Geometry: final body of the model. Coordinates: model frame, mm. Face numbers are marked on the shaded views. A direction names the side the tool comes from. Round coordinates to 2 decimals unless told otherwise and drop trailing zeros. Loops run counter-clockwise (first coordinate to the right, second up) from the corner with the lowest first, then second, coordinate; pieces in that order, holes last. Notation, with made-up numbers: (9, 36.25) - (35, 36.25) arc R31 cw to (35, 70.25) - close; hole circle Ø7 at (41.5, 45). An arc over 180 degrees is marked (long way). Answer as a JSON object with one key per item and string values. Group by question number.
Item 1: Section B-B (y = 15). Return the cut outline in (x, z), plus the area to 3 significant figures.
Item 2: Line query: line 1 (Y direction, x = -51.5, z = -28); line 2 (Z direction, x = -10, y = 16.5); line 3 (Z direction, x = -20, y = 8.5). Output: solid intervals per line, ascending.
Item 3: Section A-A (z = -27). Return the cut outline in (x, y).
Item 4: Reachability of the marked faces 1, 2 and 3 from +Z, -Z, +X, -X, +Y, -Y: full face, straight path, thin tool, end or side. Return the list, or none.
Item 5: First-contact query: pin 1 (3 mm diameter, centred on x = -67.5, z = -19.5, fed in from +Y). Flat tip, straight axial feed; report the tip coordinate or a pass-through.
Item 6: Section D-D (x = -9). Return the cut outline in (y, z).
Item 7: Section C-C (x = -65.5). Return the cut outline in (y, z), plus the area to 3 significant figures.
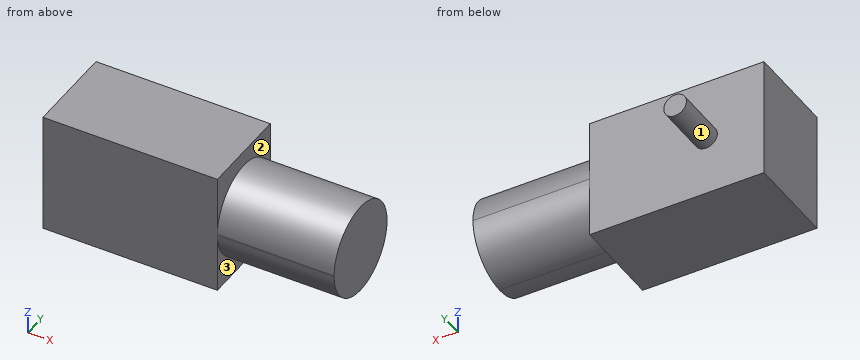
```python
from build123d import *

# Parameters (mm, degrees)
SKETCH1_W           = 76.8
SKETCH1_H           = 32
BOSS_EXTRUDE1_DEPTH = 24
SKETCH2_R           = 3
BOSS_EXTRUDE2_DEPTH = 14
CUT_EXTRUDE1_DEPTH  = 30.8


with BuildPart() as part:
    # Sketch1 → Boss-Extrude1 (new body)
    with BuildSketch(Plane(origin=(0, 0, 0), x_dir=(1, 0, 0), z_dir=(0, 1, 0))):
        with Locations((-38.4, 16)):
            Rectangle(SKETCH1_W, SKETCH1_H)
    extrude(amount=BOSS_EXTRUDE1_DEPTH)

    # Sketch2 → Boss-Extrude2 (add)
    with BuildSketch(Plane(origin=(0, 24, 0), x_dir=(1, 0, 0), z_dir=(0, 1, 0))):
        with Locations(Location((-61.466666667, 16, 0), (0, 0, 270))):
            Circle(SKETCH2_R)
    extrude(amount=BOSS_EXTRUDE2_DEPTH)

    # Sketch3 → Cut-Extrude1 (cut)
    with BuildSketch(Plane(origin=(0, 0, 0), x_dir=(0, 0, -1), z_dir=(1, 0, 0))):
        with BuildLine():
            ThreePointArc((15.826247816, 0), (3.960387057, 12.066788737), (15.960575012, 24))
            Line((15.960575012, 24), (0, 24))
            Line((0, 24), (0, 0))
            Line((0, 0), (15.826247816, 0))
        make_face()
        with BuildLine():
            Line((32, 24), (15.960575012, 24))
            ThreePointArc((15.960575012, 24), (24.446122196, 20.485171272), (27.960950924, 11.999624088))
            ThreePointArc((27.960950924, 11.999624088), (24.493481869, 3.561702389), (16.094902207, 0))
            Line((16.094902207, 0), (32, 0))
            Line((32, 0), (32, 24))
        make_face()
    extrude(amount=-CUT_EXTRUDE1_DEPTH, mode=Mode.SUBTRACT)


solid = part.part
```
Values:
{
 "1": {"outline": "(-76.8, -32) - (-30.8, -32) - (-30.8, -27.58) - (0, -27.58) - (0, -4.34) - (-30.8, -4.34) - (-30.8, 0) - (-76.8, 0) - close", "area": "2,190 mm^2"},
 "2": {"line 1": "y = 0 to 24", "line 2": "z = -27.09 to -4.84", "line 3": "z = -27.44 to -4.48"},
 "3": {"outline": "(-76.8, 0) - (-30.8, 0) - (-30.8, 7.29) - (0, 7.29) - (0, 16.7) - (-30.8, 16.7) - (-30.8, 24) - (-76.8, 24) - close"},
 "4": {"face 1": "+Y", "face 2": "+Z, +X", "face 3": "-Z, +X"},
 "5": {"pin 1": "stops at y = 24"},
 "6": {"outline": "(0, -16.09) arc R12 ccw (long way) to (0, -15.83) - close"},
 "7": {"outline": "(0, -32) - (24, -32) - (24, 0) - (0, 0) - close", "area": "768 mm^2"}
}
